Verification items for this drawing (mm, ordinates from the low corner). Give positions to 0.01 mm unless a question says otherwise; leave off trailing zeros. Loops run counter-clockwise (first coordinate to the right, second up) from the corner with the lowest first, then second, coordinate; pieces in that order, holes last. Notation, with made-up numbers: (44, 42.25) -> (76, 42.25) arc R31 ccw to (76, 70.25) -> close; hole circle Ø11 at (19.5, 55.5). An arc over 180 degrees is marked (long way). Write each question's results on one line, items separated by ' | '. Start each with the question number.
Item 1: Scan lines: line 1 along Y through (x, z) = (18.25, 5); line 2 along X through (y, z) = (2, 2); line 3 along X through (y, z) = (8.5, 3.25). Record each from-to range of solid material in increasing order.
Item 2: Gauge pin test, flat end, axial feed: pin 1 Ø1 at (y, z) = (3.5, 3) entering from +X. Record the tip position at first contact, or that the pin passes through.
Item 3: Cross-section at A-A on z = 3. Enter the section's corners in (x, y).
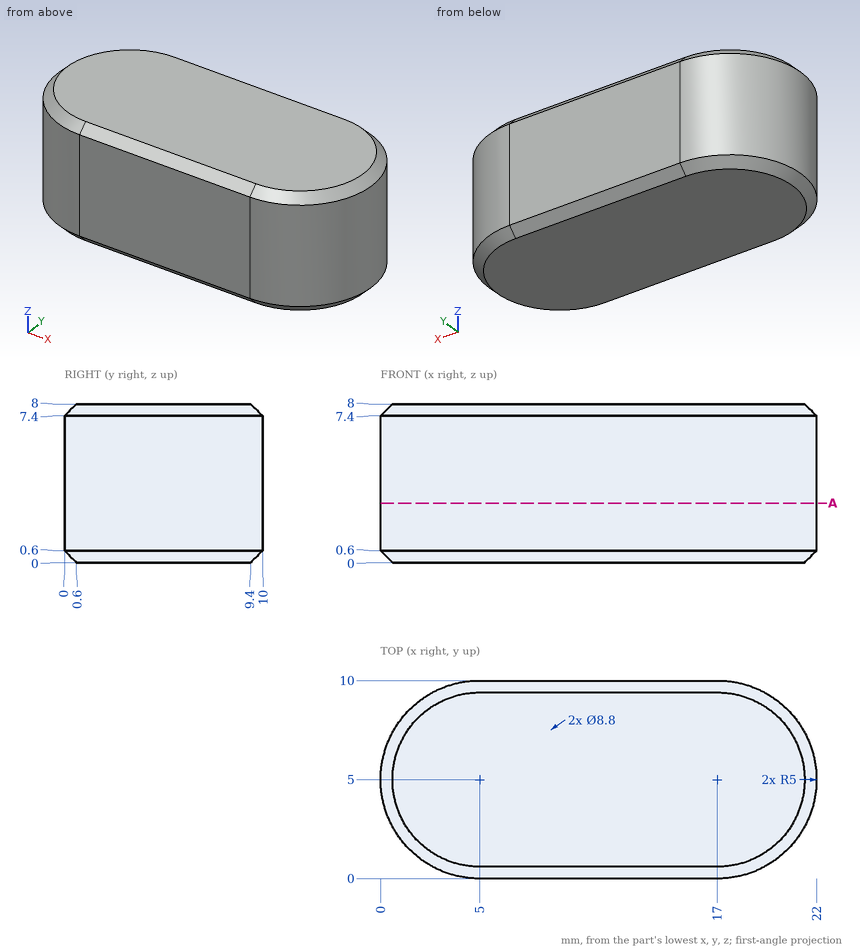
Answer sheet:
1) line 1: y = 0.16 to 9.84 | line 2: x = 1 to 21 | line 3: x = 1.43 to 20.57
2) pin 1: stops at x = 21.9
3) outline: (5, 0) -> (17, 0) arc R5 ccw to (17, 10) -> (5, 10) arc R5 ccw to start
